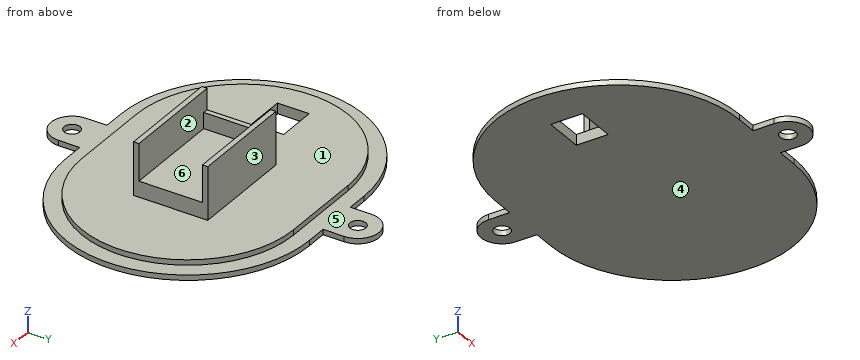
Autodesk Fusion 360 part; units mm, degrees
sketch "Sketch1" plane through (0, 0, 0) normal (0, 0, 1) x (1, 0, 0)
  line L0 (20, 0) -> (36, 0)
  line L1 (56, 20) -> (56, 20)
  line L2 (36, 40) -> (20, 40)
  line L3 (0, 20) -> (0, 20)
  arc A0 (20, 40) -> (0, 20) centre (20, 20) ccw
  arc A1 (56, 20) -> (36, 40) centre (36, 20) ccw
  arc A2 (0, 20) -> (20, 0) centre (20, 20) ccw
  arc A3 (36, 0) -> (56, 20) centre (36, 20) ccw
  point P0 (55, 0)
  point P1 (0, 40)
  dimension "d1" = 55
  dimension "d2" = 40
  dimension "d3" = 20
  dimension "d4" = 20
  dimension "d5" = 20
  dimension "d6" = 20
extrude "Extrude1" add sketch "Sketch1" along normal blind 1
sketch "Sketch2" plane through (0, 0, 0) normal (0, 0, -1) x (1, 0, 0)
  arc A0 (36, -40) -> (36, 0) centre (36, -20) ccw
  line L0 (36, 0) -> (20, 0)
  arc A1 (20, 0) -> (20, -40) centre (20, -20) ccw
  line L1 (20, -40) -> (36, -40)
  arc A2 (36, -43) -> (36, 3) centre (36, -20) ccw
  line L2 (36, 3) -> (20, 3)
  arc A3 (20, 3) -> (20, -43) centre (20, -20) ccw
  line L3 (20, -43) -> (36, -43)
  line L4 (28, 0) -> (28, 8) construction
  line L5 (28, 0) -> (24, 0) construction
  line L6 (24, 0) -> (32, 0)
  line L7 (32, 0) -> (32, 7)
  line L8 (28, 11) -> (28, 11)
  line L9 (24, 7) -> (24, 0)
  arc A4 (28, 11) -> (24, 7) centre (28, 7) ccw
  arc A5 (32, 7) -> (28, 11) centre (28, 7) ccw
  line L10 (0, -20) -> (56, -20)
  line L11 (28, -40) -> (28, -48) construction
  line L12 (28, -40) -> (32, -40)
  line L13 (32, -40) -> (24, -40)
  line L14 (24, -40) -> (24, -47)
  line L15 (28, -51) -> (28, -51)
  line L16 (32, -47) -> (32, -40)
  arc A6 (24, -47) -> (28, -51) centre (28, -47) ccw
  arc A7 (28, -51) -> (32, -47) centre (28, -47) ccw
  circle A8 centre (28, 7) radius 1.5
  circle A9 centre (28, -47) radius 1.5
  point P0 (24, 11)
  point P1 (32, -51)
  dimension "d9" = 3
  dimension "d12" = 8
  dimension "d13" = 4
  dimension "d14" = 8
  dimension "d15" = 11
  dimension "d16" = 4
  dimension "d17" = 4
  dimension "d18" = 8
  dimension "d19" = 4
  dimension "d20" = 8
  dimension "d21" = 11
  dimension "d22" = 4
  dimension "d23" = 4
  dimension "d26" = 3
  dimension "d27" = 3
extrude "Extrude2" add sketch "Sketch2" along normal blind 1 contours A0 A1 L1 L10 L12 L13 | A0 L0 L1 A2 L2 L3 L7 L16 | A0 L0 A1 L6 L10 | L1 L3 L12 L13 L14 L16 | L0 A1 L1 L2 A3 L3 L9 L14 | L0 L2 L6 L7 L9
extrude "Extrude3" add sketch "Sketch2" along normal up to surface (1 mm away) contours L3 L14 L16 A6 A7 | L2 L7 L9 A4 A5 | A8 | A9
extrude "Extrude4" cut sketch "Sketch2" along normal up to surface (1 mm away) contours A8 | A9
sketch "Sketch3" plane through (0, 0, 1) normal (0, 0, 1) x (-1, 0, 0)
  arc A0 (-36, 0) -> (-36, -40) centre (-36, -20) ccw
  line L0 (-36, -40) -> (-20, -40)
  arc A1 (-20, -40) -> (-20, 0) centre (-20, -20) ccw
  line L1 (-20, 0) -> (-36, 0)
  line L2 (0, -20) -> (-56, -20)
  line L3 (-21, -20) -> (-21, -26) construction
  line L4 (-21, -26) -> (-22, -26)
  line L5 (-22, -26) -> (-22, -14)
  line L6 (-22, -14) -> (-21, -14)
  line L7 (-21, -14) -> (-21, -26)
  line L8 (-21, -27) -> (-41, -27)
  line L9 (-41, -27) -> (-41, -26)
  line L10 (-41, -26) -> (-21, -26)
  line L11 (-21, -26) -> (-21, -27)
  line L12 (-21, -14) -> (-41, -14)
  line L13 (-41, -14) -> (-41, -13)
  line L14 (-41, -13) -> (-21, -13)
  line L15 (-21, -13) -> (-21, -14)
  line L16 (-5, -23) -> (-12.5, -23)
  line L17 (-12.5, -23) -> (-12.5, -17)
  line L18 (-12.5, -17) -> (-5, -17)
  line L19 (-5, -17) -> (-5, -23)
  line L20 (-22, -26) -> (-41, -26)
  line L21 (-41, -26) -> (-41, -14)
  line L22 (-41, -14) -> (-22, -14)
  line L23 (-22, -14) -> (-22, -26)
  dimension "d34" = 6
  dimension "d35" = 1
  dimension "d36" = 12
  dimension "d37" = 20
  dimension "d38" = 20
  dimension "d44" = 7.5
  dimension "d45" = 6
extrude "Extrude5" add sketch "Sketch3" along normal blind 6 contours L2 L5 L6 L7 L12 L23 | L2 L4 L5 L7 L10 L23
extrude "Extrude6" add sketch "Sketch3" along normal blind 10 contours L4 L8 L9 L10 L11 L20 | L6 L12 L13 L14 L15 L22
extrude "Extrude7" cut sketch "Sketch3" against normal up to surface (2 mm away) contours L2 L16 L17 L19 | L2 L17 L18 L19
extrude "Extrude8" add sketch "Sketch3" along normal blind 3 contours L2 L5 L12 L21 L22 L23 | L2 L5 L10 L20 L21 L23
Build history of the part. All positions in model axes, mm. Face numbers are marked on the shaded views. A direction names the side the tool comes from. Give positions to 0.01 mm unless a question says otherwise; leave off trailing zeros. Loops run counter-clockwise (first coordinate to the right, second up) from the corner with the lowest first, then second, coordinate; pieces in that order, holes last.
Item 1: Slice it at B-B, the plane z = 8.25. List the corners of the cut face in (x, y), and give its area (3 significant figures).
Answers follow:
outline: (21, 13) - (41, 13) - (41, 14) - (21, 14) - close; (21, 26) - (41, 26) - (41, 27) - (21, 27) - close
area: 40.0 mm2
Item 2: Drill centre lines: line 1 (Y direction, x = 28, z = -0.8); line 2 (X direction, y = 47, z = -0.3); line 3 (Y direction, x = 21.5, z = 9.25). Where is each one in solid material? Low to high.
Answers follow:
line 1: y = -11 to -8.5, -5.5 to 45.5, 48.5 to 51
line 2: x = 24 to 26.5, 29.5 to 32
line 3: y = 13 to 14, 26 to 27
Item 3: Flat gauge pins, fed straight in: pin 1 (0.8 mm diameter, centred on x = 33.5, z = -0.5, fed in from -Y); pin 2 (6 mm diameter, centred on x = 5.5, z = 6, fed in from -Y); pin 3 (2 mm diameter, centred on y = 20, z = 0, fed in from -X); pin 4 (2 mm diameter, centred on x = 22.5, z = 6, fed in from +Y). Where does each tip first touch, or does it go through?
Answers follow:
pin 1: stops at y = -3
pin 2: passes through
pin 3: stops at x = -3
pin 4: stops at y = 27
Item 4: Slice it at A-A, the plane y = 20. List the corners of the cut face in (x, z), and give its area (3 significant figures).
Answers follow:
outline: (-3, -1) - (5, -1) - (5, 1) - (0, 1) - (0, 0) - (-3, 0) - close; (12.5, -1) - (59, -1) - (59, 0) - (56, 0) - (56, 1) - (41, 1) - (41, 4) - (22, 4) - (22, 7) - (21, 7) - (21, 1) - (12.5, 1) - close
area: 166 mm2
Item 5: Slice it at D-D, the plane x = 8. List the corners of the cut face in (y, z), and give its area (3 significant figures).
Answers follow:
outline: (0.38, -1) - (17, -1) - (17, 1) - (4, 1) - (4, 0) - (0.38, 0) - close; (23, -1) - (39.62, -1) - (39.62, 0) - (36, 0) - (36, 1) - (23, 1) - close
area: 59.2 mm2
Item 6: Which spindle directions (+Z, -Z, +X, -X, +Y, -Y) get a long thin tool onto all of the face, cutting with end or side? Do the marked faces 4, 5 and 6. Say none if no direction does.
Answers follow:
face 4: -Z, +X, -X, +Y, -Y
face 5: +Z
face 6: +Z, +X
Item 7: Slice it at C-C, the plane x = 28. List the corners of the cut face in (y, z), and give its area (3 significant figures).
Answers follow:
outline: (-11, -1) - (-8.5, -1) - (-8.5, 0) - (-11, 0) - close; (-5.5, -1) - (45.5, -1) - (45.5, 0) - (40, 0) - (40, 1) - (27, 1) - (27, 11) - (26, 11) - (26, 4) - (14, 4) - (14, 11) - (13, 11) - (13, 1) - (0, 1) - (0, 0) - (-5.5, 0) - close; (48.5, -1) - (51, -1) - (51, 0) - (48.5, 0) - close
area: 152 mm2
Item 8: Pull direction Y, two halves, no side cores. Call the marked faces 1, 2 and 3: released by +Y, released by -Y, zero draft, split by the parting line, or undercut.
Answers follow:
face 1: zero draft
face 2: undercut
face 3: released by +Y
